The listing builds one solid part. Answer for the finished solid, in the listing's coordinates (mm). A direction names the side the tool comes from. Coordinates: 2 decimals unless noted, no trailing zeros. Write each loop counter-clockwise with the first axis right and the second up, starting at its lowest first coordinate (ties: lowest second). Pieces come first, ordered by that corner, then holes. Notation, with made-up numbers: M -12.5,66.25 L 25.5,66.25 A18 ccw 25.5,87.25 Z; hole C -10,-3 d5. An arc over 180 degrees is marked long. Answer as CSV lines item,"result".
```python
from build123d import *

# Parameters (mm, degrees)
SKETCH_W        = 40
SKETCH_H        = 85
PAD_DEPTH       = 50
POCKET_DEPTH    = 50
POCKET001_DEPTH = 20
SKETCH003_W     = 16
SKETCH003_H     = 26
POCKET002_DEPTH = 18
SKETCH004_R     = 2
POCKET003_DEPTH = 4
SKETCH005_R     = 2
POCKET004_DEPTH = 4
POCKET005_DEPTH = 2
SKETCH007_W     = 34
SKETCH007_H     = 60
POCKET006_DEPTH = 32
SKETCH008_R     = 4.5
SKETCH008_R_2   = 5.95
POCKET007_DEPTH = 18
SKETCH009_R     = 10.85
POCKET008_DEPTH = 8
POCKET009_DEPTH = 40.001


with BuildPart() as part:
    # Sketch → Pad (new body)
    with BuildSketch(Plane.YZ):
        Rectangle(SKETCH_W, SKETCH_H)
    extrude(amount=PAD_DEPTH)

    # Sketch001 (on Face6 of Pad) → Pocket (cut)
    with BuildSketch(Plane.YZ.offset(50)):
        Polygon((-20, -22.5), (-20, -42.5), (0, -42.5), (0, -22.5), (-7.51604, -22.5), (-7.51604, -24.5), (-4.81604, -24.5), (-8, -27.68), (-12, -27.68), (-15.18396, -24.5), (-12.48396, -24.5), (-12.48396, -22.5), align=None)
    extrude(amount=-POCKET_DEPTH, mode=Mode.SUBTRACT)

    # Sketch002 (on Face3 of Pocket) → Pocket001 (cut)
    with BuildSketch(Plane.ZX.offset(20)):
        Polygon((-22.5, 50), (-42.5, 50), (-42.5, 30), (-22.5, 30), (-22.5, 37.52), (-24.5, 37.52), (-24.5, 34.82), (-27.68, 38), (-27.68, 42), (-24.5, 45.18), (-24.5, 42.48), (-22.5, 42.48), align=None)
    extrude(amount=-POCKET001_DEPTH, mode=Mode.SUBTRACT)

    # Sketch003 (on Face3 of Pocket001) → Pocket002 (cut)
    with BuildSketch(Plane.ZX.offset(20)):
        with Locations((-32.5, 13)):
            Rectangle(SKETCH003_W, SKETCH003_H)
    extrude(amount=-POCKET002_DEPTH, mode=Mode.SUBTRACT)

    # Sketch004 (on Face30 of Pocket002) → Pocket003 (cut)
    with BuildSketch(Plane.ZX.offset(2)):
        with Locations((-32.5, 13)):
            Circle(SKETCH004_R)
    extrude(amount=-POCKET003_DEPTH, mode=Mode.SUBTRACT)

    # Sketch005 (on Face8 of Pocket003) → Pocket004 (cut)
    with BuildSketch(Plane(origin=(26, 0, 0), x_dir=(0, 1, 0), z_dir=(-1, 0, 0))):
        with Locations((11, 32.5)):
            Circle(SKETCH005_R)
    extrude(amount=-POCKET004_DEPTH, mode=Mode.SUBTRACT)

    # Sketch006 (on Face10 of Pocket004) → Pocket005 (cut)
    with BuildSketch(Plane.YX.offset(42.5)):
        Polygon((2.005691, 0), (20, 26), (20, 0), align=None)
    extrude(amount=-POCKET005_DEPTH, mode=Mode.SUBTRACT)

    # Sketch007 (on Face5 of Pocket005) → Pocket006 (cut)
    with BuildSketch(Plane.YZ.offset(50)):
        with Locations((0, 12.5)):
            Rectangle(SKETCH007_W, SKETCH007_H)
    extrude(amount=-POCKET006_DEPTH, mode=Mode.SUBTRACT)

    # Sketch008 (on Face6 of Pocket006) → Pocket007 (cut)
    with BuildSketch(Plane.YZ.offset(18)):
        with Locations((0, 3.5)):
            Circle(SKETCH008_R)
        with Locations((0, 25.5)):
            Circle(SKETCH008_R_2)
    extrude(amount=-POCKET007_DEPTH, mode=Mode.SUBTRACT)

    # Sketch009 (on Face2 of Pocket007) → Pocket008 (cut)
    with BuildSketch(Plane(origin=(0, 0, 0), x_dir=(0, 1, 0), z_dir=(-1, 0, 0))):
        with Locations((0, -3.5)):
            Circle(SKETCH009_R)
    extrude(amount=-POCKET008_DEPTH, mode=Mode.SUBTRACT)

    # Sketch010 (on Face3 of Pocket008) → Pocket009 (cut, through all)
    with BuildSketch(Plane.ZX.offset(20)):
        Polygon((-17.5, 50), (42.5, 50), (42.5, 25), align=None)
    extrude(amount=-POCKET009_DEPTH, mode=Mode.SUBTRACT)


solid = part.part
```
Q1. For faces 1 (the flat face through (12.82, 10.88, -41.51)), 2 (the flat face through (31, 17, 5)), 3 (the flat face through (31, 3, -22.5)), 4 (the flat face through (25, -7.516, -23)), determine the directions among +Z, -Z, +X, -X, +Y, -Y from which every point of the face is accessible in a straight line to the end or side of a thin tool.
Output:
face 1,"-Z, -X, +Y"
face 2,"+Z, +X"
face 3,"none"
face 4,"+X, -X"
Q2. Find section D-D (z = 25.5). Give the vertices of the cut face in (x, y).
Output:
outline,"M 0,-20 L 32.08,-20 L 32.08,-17 L 18,-17 L 18,-5.95 L 0,-5.95 Z; M 0,5.95 L 18,5.95 L 18,17 L 32.08,17 L 32.08,20 L 0,20 Z"
Q3. Straight lines are drawn through the part: line 1 (Y direction, x = 29.15, z = -32.5); line 2 (Y direction, x = 3.5, z = 3.5); line 3 (X direction, y = 11, z = 39). For each, find the intervals that lie inside material, in ascending order.
Output:
line 1,"0 to 9, 13 to 20"
line 2,"-20 to -10.85, 10.85 to 20"
line 3,"0 to 18"
Q4. Find section C-C (x = 33). Give the vertices of the cut face in (y, z).
Output:
outline,"M -20,-22.5 L -12.48,-22.5 L -12.48,-24.5 L -15.18,-24.5 L -12,-27.68 L -8,-27.68 L -4.82,-24.5 L -7.52,-24.5 L -7.52,-22.5 L 20,-22.5 L 20,23.3 L 17,23.3 L 17,-17.5 L -17,-17.5 L -17,23.3 L -20,23.3 Z"
Q5. Find section B-B (z = -32.5). Give the vertices of the cut face in (x, y), and give its area (3 significant figures).
Output:
outline,"M 0,0 L 11,0 L 11,2 L 0,2 Z; M 15,0 L 30,0 L 30,9 L 26,9 L 26,2 L 15,2 Z; M 26,13 L 30,13 L 30,20 L 26,20 Z"
area,"108 mm2"
Q6. The mould has two halves that part along Z. Classify faces 5 (the flat face through (15.2, 0, -32.6)), 6 (the flat face through (34, 0, -17.5)), 7 (the flat face through (25, -16, -22.5)): pulls with the +Z half, pulls with the -Z half, needs draft (parallel to the pull), parting line crosses it, or undercut.
Output:
face 5,"needs draft"
face 6,"pulls with the +Z half"
face 7,"undercut"
Q7. Flat-ended cylindrical pins translate along their axes: pin 1 Ø12 at (x, y) = (38, 4) entering from -Z; pin 2 Ø6.5 at (y, z) = (11, -32.5) entering from +X; pin 3 Ø5.5 at (y, z) = (0, 3.5) entering from -X; pin 4 Ø2 at (y, z) = (11, 5) entering from +X. Find the tip coordinate at first contact, or state that the pin passes through.
Output:
pin 1,"z = -27.68"
pin 2,"x = 30"
pin 3,"through"
pin 4,"x = 18"
Q8. Find section A-A (x = 13). Give the vertices of the cut face in (y, z).
Output:
outline,"M -20,-22.5 L -12.48,-22.5 L -12.48,-24.5 L -15.18,-24.5 L -12,-27.68 L -8,-27.68 L -4.82,-24.5 L -7.52,-24.5 L -7.52,-22.5 L 0,-22.5 L 0,-30.5 L 2,-30.5 L 2,-24.5 L 20,-24.5 L 20,42.5 L -20,42.5 Z; M 0,-42.5 L 11,-42.5 L 11,-40.5 L 2,-40.5 L 2,-34.5 L 0,-34.5 Z; hole C 0,25.5 d11.9; hole C 0,3.5 d9"
